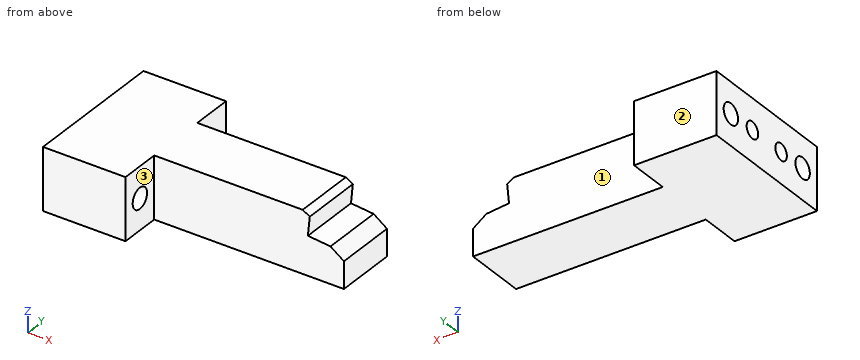
from build123d import *

# Parameters (mm, degrees)
F0_W     = 20
F0_H     = 7.5
F1_DEPTH = 35
F2_W     = 35.998606
F2_H     = 10
F2_W_2   = 10.001394
F3_DEPTH = 15.001
F4_R     = 2.5
F5_DEPTH = 20.001
F6_R     = 2
F7_DEPTH = 6


with BuildPart() as f1:
    # F0 (on Front) → F1 (new body)
    with BuildSketch(Plane.XZ):
        with Locations((-67.633515, -45.922072)):
            Rectangle(F0_W, F0_H)
        with Locations((-67.633515, -38.422072)):
            Rectangle(F0_W, F0_H)
        Polygon((-11.633515, -49.672072), (-11.633515, -43.181855), (-14.883661, -40.850213), (-20.370748, -40.306831), (-19.911289, -35.667204), (-21.634909, -34.672072), (-57.633515, -34.672072), (-57.633515, -42.172072), (-57.633515, -49.672072), align=None)
    extrude(amount=F1_DEPTH)

    # F2 (on face) → F3 (cut, through all)
    with BuildSketch(Plane.XY.offset(-34.672072)):
        with Locations((-39.634212, -5)):
            Rectangle(F2_W, F2_H)
        with Locations((-16.634212, -30)):
            Rectangle(F2_W_2, F2_H)
        with Locations((-16.634212, -5)):
            Rectangle(F2_W_2, F2_H)
        with Locations((-39.634212, -30)):
            Rectangle(F2_W, F2_H)
    extrude(amount=-F3_DEPTH, mode=Mode.SUBTRACT)

    # F4 (on face) → F5 (cut, through all)
    with BuildSketch(Plane.YZ.offset(-57.633515)):
        with Locations((-30, -42.172072)):
            Circle(F4_R)
        with Locations((-5, -42.172072)):
            Circle(F4_R)
    extrude(amount=-F5_DEPTH, mode=Mode.SUBTRACT)

    # F6 (on face) → F7 (cut)
    with BuildSketch(Plane(origin=(-77.633515, 0, 0), x_dir=(0, -1, 0), z_dir=(-1, 0, 0))):
        with Locations((12.5, -42.172072)):
            Circle(F6_R)
        with Locations((22.5, -42.172072)):
            Circle(F6_R)
    extrude(amount=-F7_DEPTH, mode=Mode.SUBTRACT)


solid = f1.part
CAD build for the part. Positions are in the model's coordinates, mm. Face numbers are marked on the shaded views. A direction names the side the tool comes from. Coordinates: 2 decimals unless noted, no trailing zeros. Write each loop counter-clockwise with the first axis right and the second up, starting at its lowest first coordinate (ties: lowest second). Pieces come first, ordered by that corner, then holes. Notation, with made-up numbers: M -25.75,10 L 28.25,10 A26 ccw 28.25,38 Z; hole C 18,29.5 d9. An arc over 180 degrees is marked long. Answer as a JSON object with one key per item and string values. Group by question number.
1) Saw through at D-D (x = -42). Write the cut outline in (y, z).
2) Wall check: line 1 (Z direction, x = -62.5, y = -5); line 2 (Z direction, x = -76.15, y = -12.5); line 3 (Y direction, x = -65.5, z = -42.75). Give the ranges that are in metal, low to high. Write a range as from..to.
3) Saw through at A-A (y = -5). Write the cut outline in (x, z), plus the area to 3 significant figures.
4) Saw through at B-B (y = -12.5). Write the cut outline in (x, z), plus the area to 3 significant figures.
5) Tool access for the marked faces 1, 2 and 3: list every direction of +Z, -Z, +X, -X, +Y, -Y with a clear straight run to the whole face (end or side of a thin tool).
6) Pin check, flat tips, straight feed: pin 1 Ø1 at (x, z) = (-47.5, -41) entering from -Y; pin 2 Ø8 at (x, z) = (-44, -45.5) entering from +Y; pin 3 Ø4 at (y, z) = (-30.5, -48) entering from +X. Stop position of each tip, or through.
7) Saw through at C-C (z = -46.75). Write the cut outline in (x, y), plus the area to 3 significant figures.
Values follow:
{
 "1": {"outline": "M -25,-49.67 L -10,-49.67 L -10,-34.67 L -25,-34.67 Z"},
 "2": {"line 1": "z = -49.67..-44.67, -39.67..-34.67", "line 2": "z = -49.67..-44.17, -40.17..-34.67", "line 3": "y = -35..-32.43, -27.57..-7.43, -2.57..0"},
 "3": {"outline": "M -77.63,-49.67 L -57.63,-49.67 L -57.63,-44.67 L -77.63,-44.67 Z; M -77.63,-39.67 L -57.63,-39.67 L -57.63,-34.67 L -77.63,-34.67 Z", "area": "200 mm2"},
 "4": {"outline": "M -77.63,-49.67 L -11.63,-49.67 L -11.63,-43.18 L -14.88,-40.85 L -20.37,-40.31 L -19.91,-35.67 L -21.63,-34.67 L -77.63,-34.67 L -77.63,-40.17 L -71.63,-40.17 L -71.63,-44.17 L -77.63,-44.17 Z", "area": "910 mm2"},
 "5": {"face 1": "+Z, -Z, +X, +Y", "face 2": "+Z, -Z, +X, -X, +Y", "face 3": "+Z, -Z, +X, -Y"},
 "6": {"pin 1": "stops at y = -25", "pin 2": "stops at y = -10", "pin 3": "stops at x = -57.63"},
 "7": {"outline": "M -77.63,-35 L -57.63,-35 L -57.63,-25 L -11.63,-25 L -11.63,-10 L -57.63,-10 L -57.63,0 L -77.63,0 Z", "area": "1,390 mm2"}
}
